Autodesk Inventor part; units mm, degrees
ref_plane "YZ Plane" through (0, 0, 0) normal (1, 0, 0) x (0, 1, 0)
ref_plane "XZ Plane" through (0, 0, 0) normal (0, 1, 0) x (-1, 0, 0)
ref_plane "XY Plane" through (0, 0, 0) normal (0, 0, 1) x (1, 0, 0)
sketch "Sketch1" plane through (0, 0, 0) normal (0, 1, 0) x (-1, 0, 0)
  circle A0 centre (0, 0) radius 15.875
  circle A1 centre (0, 0) radius 50.8
  line L0 (0, -50.8) -> (133.35, -50.8)
  line L1 (133.35, -50.8) -> (133.35, 6.35)
  line L2 (133.35, 6.35) -> (56.3603, 50.8)
  line L3 (56.3603, 50.8) -> (0, 50.8)
  circle A2 centre (82.55, -19.05) radius 9.525
  dimension "d0" = 101.6
  dimension "d1" = 133.35
  dimension "d4" = 60
  dimension "d5" = 57.15
  dimension "d6" = 31.75
  dimension "d7" = 19.05
  dimension "d8" = 31.75
  dimension "d9" = 82.55
extrude "MAIN BLOCK" add sketch "Sketch1" along normal blind 63.5
sketch "Sketch2" plane through (0, 63.5, 0) normal (0, 1, 0) x (1, 0, 0)
  line L0 (-31.75, -50.8) -> (50.8, -50.8)
  line L1 (50.8, -50.8) -> (50.8, 50.8)
  line L2 (50.8, 50.8) -> (-31.75, 50.8)
  line L3 (-31.75, 50.8) -> (-31.75, -50.8)
  arc A0 (0, -50.8) -> (0, 50.8) centre (0, 0) ccw
  line L4 (0, 50.8) -> (-133.35, 50.8)
  line L5 (-56.3603, -50.8) -> (0, -50.8)
  point P0 (0, 50.8)
  dimension "d12" = 31.75
extrude "SQUARE CUTOUT" cut sketch "Sketch2" against normal blind 38.1 contours L3 L2 A0 L0
sketch "Sketch3" plane through (0, 63.5, 0) normal (0, 1, 0) x (1, 0, 0)
  line L0 (-31.75, -50.8) -> (-31.75, 50.8)
  circle A0 centre (-31.75, 0) radius 31.75
  point P0 (0, 0)
  point P1 (-31.75, 31.75)
  point P2 (-31.75, -31.75)
  dimension "d15" = 63.5
extrude "HALF CIRCLE CUTOUT" cut sketch "Sketch3" against normal blind 19.05 contours A0 L0 picked at (-42.2562, -1.2757)
chamfer "REAR CHAMFER" distance 25.4 angle 45 1 edges at (-133.35, 63.5, -22.225)
properties part number "ANS8-2-BK" material "Bronze, Cast"
Part model, mm, in its own coordinate system. A direction names the side the tool comes from. Give positions to 0.01 mm unless a question says otherwise; leave off trailing zeros. Order: outer loops, then holes, each group sorted by start corner. A loop starts at its lowest first (then second) coordinate and runs counter-clockwise, first axis right, second up. Notation, with made-up numbers: (-36.5, 75.5) -> (-16.5, 75.5) arc R20 ccw to (-16.5, 81.5) -> close; hole circle Ø6 at (-2.75, 49.5). An arc over 180 degrees is marked (long way). Use one line per item in the form item = value.
(1) Saw through at C-C (z = -19.05). Write the cut outline in (x, y) (3 decimals).
Solution:
outline = (-133.35, 0) -> (-92.075, 0) -> (-92.075, 63.5) -> (-107.95, 63.5) -> (-133.35, 38.1) -> close; (-73.025, 0) -> (47.093, 0) -> (47.093, 25.4) -> (-31.75, 25.4) -> (-31.75, 44.45) -> (-57.15, 44.45) -> (-57.15, 63.5) -> (-73.025, 63.5) -> close
(2) Drill centre lines: line 1 (Z direction, x = 0, y = 17.5) (3 decimals); line 2 (X direction, y = 38, z = -19); line 3 (Y direction, x = 20, z = 37). Where is each one in solid material? Low to high. Write a range as from..to.
Solution:
line_1 = -50.8..-15.875, 15.875..50.8
line_2 = -133.35..-92.07, -73.03..-31.75
line_3 = 0..25.4
(3) Pull direction X, two halves, no side cores. Call faces 1 (the face through (3.441, 12.522, 15.497)), 2 (the face through (-120.47, 50.98, -14.39)), 3 (the face through (18, 25.4, -1)): +X half, -X half, draft (parallel to the pull), parting line (faces both ways), or undercut.
Solution:
face_1 = undercut
face_2 = -X half
face_3 = draft
(4) Flat gauge pins, fed straight in: P1, Ø3, axis at y = 53, z = 2, coming from the +X side; P2, Ø8, axis at x = 7.5, z = -33.5, coming from the +Y side; P3, Ø8, axis at x = 17.5, y = 27.5, coming from the -Z side. Where does each tip first touch, or does it go through?
Solution:
P1 = -63.31
P2 = 25.4
P3 = -48.81
(5) Tool access for faces 4 (the face through (-95.394, 31.306, 28.264)), 5 (the face through (-63.492, 54.108, -0.698)), 6 (the face through (-31.75, 40, -1)): list every direction of +Z, -Z, +X, -X, +Y, -Y with a clear straight run to the whole face (end or side of a thin tool).
Solution:
face_4 = +Z, -X, +Y, -Y
face_5 = +X, +Y
face_6 = +Z, -Z, +X, +Y
(6) Saw through at B-B (x = -82.55). Write the cut outline in (y, z) (3 decimals).
Solution:
outline = (0, -50.8) -> (63.5, -50.8) -> (63.5, -28.575) -> (0, -28.575) -> close; (0, -9.525) -> (63.5, -9.525) -> (63.5, 35.679) -> (0, 35.679) -> close
(7) Saw through at D-D (z = 25). Write the cut outline in (x, y), then the cut area to 3 significant figures.
Solution:
outline = (-101.05, 0) -> (44.22, 0) -> (44.22, 25.4) -> (-31.75, 25.4) -> (-31.75, 44.45) -> (-51.32, 44.45) -> (-51.32, 63.5) -> (-101.05, 63.5) -> close
area = 5,960 mm²
(8) Saw through at A-A (y = 23). Write the cut outline in (x, z) (3 decimals).
Solution:
outline = (-133.35, -50.8) -> (0, -50.8) arc R50.8 ccw to (0, 50.8) -> (-56.36, 50.8) -> (-133.35, 6.35) -> close; hole circle Ø19.05 at (-82.55, -19.05); hole circle Ø31.75 at (0, 0)
